Design review of the part built by this model. Coordinates are the model's own, in mm. A direction names the side the tool comes from. Give positions to 0.01 mm unless a question says otherwise; leave off trailing zeros. Order: outer loops, then holes, each group sorted by start corner. A loop starts at its lowest first (then second) coordinate and runs counter-clockwise, first axis right, second up. Notation, with made-up numbers: M 77,30.25 L 95,30.25 A11 cw 95,50.25 Z; hole C 12.5,20.25 d11. An arc over 180 degrees is marked long. Answer as a JSON object with one key per item and string values.
from build123d import *
from build123d.topology import SkipClean

# Parameters (mm, degrees)
SKETCH2_R           = 3.556
BOSS_EXTRUDE1_DEPTH = 0.254
CUT_EXTRUDE1_DEPTH  = 15.202896108
CUT_EXTRUDE2_DEPTH  = 15.331771344
FILLET1_R           = 0.396875


with BuildPart() as part:
    # Sketch1 → Base-Revolve (revolve)
    with BuildSketch(Plane.XY, mode=Mode.PRIVATE) as base_revolve_sk:
        Polygon((7.112, 0), (7.112, 8.69315), (5.08, 8.69315), (5.08, 8.1153), (3.556, 8.1153), (0, 8.1153), (0, 0), align=None)
    revolve(base_revolve_sk.sketch.rotate(Axis((0, 0, 0), (1, 0, 0)), 90), axis=Axis((0, 0, 0), (1, 0, 0)))

    # Sketch2 → Boss-Extrude1 (add)
    with BuildSketch(Plane(origin=(7.112, 0, 0), x_dir=(0, 0, -1), z_dir=(1, 0, 0))):
        with Locations(Location((0, 0, 0), (0, 0, 180))):
            Circle(SKETCH2_R)
    extrude(amount=BOSS_EXTRUDE1_DEPTH)

    # Sketch3 → Cut-Extrude1 (cut, through all)
    with SkipClean():  # the faces are left unmerged after this step: merging them gives an invalid solid
        with BuildSketch(Plane(origin=(7.112, 0, 0), x_dir=(0, 0, -1), z_dir=(1, 0, 0))):
            with BuildLine():
                ThreePointArc((2.61585906, -5.29454546), (5.9055, 0), (2.61585906, 5.29454546))
                ThreePointArc((2.61585906, 5.29454546), (1.042283968, 4.761688488), (1.57514094, 3.188113395))
                ThreePointArc((1.57514094, 3.188113395), (3.556, 0), (1.57514094, -3.188113395))
                ThreePointArc((1.57514094, -3.188113395), (1.042283968, -4.761688488), (2.61585906, -5.29454546))
            make_face()
            with BuildLine():
                ThreePointArc((-2.61585906, -5.29454546), (-1.042283968, -4.761688488), (-1.57514094, -3.188113395))
                ThreePointArc((-1.57514094, -3.188113395), (-3.556, 0), (-1.57514094, 3.188113395))
                ThreePointArc((-1.57514094, 3.188113395), (-1.042283968, 4.761688488), (-2.61585906, 5.29454546))
                ThreePointArc((-2.61585906, 5.29454546), (-5.9055, 0), (-2.61585906, -5.29454546))
            make_face()
        extrude(amount=-CUT_EXTRUDE1_DEPTH, mode=Mode.SUBTRACT)

    # Sketch4 → Cut-Extrude2 (cut, through all)
    with SkipClean():  # the faces are left unmerged after this step: merging them gives an invalid solid
        with BuildSketch(Plane(origin=(7.366, 0, 0), x_dir=(0, 0, -1), z_dir=(1, 0, 0))):
            with BuildLine():
                Line((3.434727855, 0.92075), (0.92075, 0.92075))
                Line((0.92075, 0.92075), (0.92075, 2.202919244))
                ThreePointArc((0.92075, 2.202919244), (0, 2.3876), (-0.92075, 2.202919244))
                Line((-0.92075, 2.202919244), (-0.92075, 0.92075))
                Line((-0.92075, 0.92075), (-3.434727855, 0.92075))
                ThreePointArc((-3.434727855, 0.92075), (-3.556, 0), (-3.434727855, -0.92075))
                Line((-3.434727855, -0.92075), (-0.92075, -0.92075))
                Line((-0.92075, -0.92075), (-0.92075, -2.202919244))
                ThreePointArc((-0.92075, -2.202919244), (0, -2.3876), (0.92075, -2.202919244))
                Line((0.92075, -2.202919244), (0.92075, -0.92075))
                Line((0.92075, -0.92075), (3.434727855, -0.92075))
                ThreePointArc((3.434727855, -0.92075), (3.556, 0), (3.434727855, 0.92075))
            make_face()
        extrude(amount=-CUT_EXTRUDE2_DEPTH, mode=Mode.SUBTRACT)

    # Fillet1
    fillet1_edges = [part.edges().sort_by_distance(p)[0] for p in [
        (3.683, -0.92075, -0.92075),
        (3.683, -0.92075, 0.92075),
        (3.683, 0.92075, 0.92075),
        (3.683, 0.92075, -0.92075),
    ]]
    fillet(fillet1_edges, radius=FILLET1_R)

    # Boss-Mirror1: part across face


with BuildPart() as part_1:
    with SkipClean():  # the faces are left unmerged after this step: merging them gives an invalid solid
        add(part.part)
        add(part.part.mirror(Plane.ZY))


solid = part_1.part
(1) We need section C-C (x = -2). Write out the cut boundary in (y, z), plus the area to 3 significant figures.
Checked values:
{"outline": "C 0,0 d16.23; hole M -5.29,-2.62 A5.91 ccw 5.29,-2.62 A1.17 ccw 3.19,-1.58 A3.56 cw 0.92,-3.43 L 0.92,-1.32 A0.4 cw 1.32,-0.92 L 2.2,-0.92 A2.39 ccw 2.2,0.92 L 1.32,0.92 A0.4 cw 0.92,1.32 L 0.92,3.43 A3.56 cw 3.19,1.58 A1.17 ccw 5.29,2.62 A5.91 ccw -5.29,2.62 A1.17 ccw -3.19,1.58 A3.56 cw -0.92,3.43 L -0.92,1.32 A0.4 cw -1.32,0.92 L -2.2,0.92 A2.39 ccw -2.2,-0.92 L -1.32,-0.92 A0.4 cw -0.92,-1.32 L -0.92,-3.43 A3.56 cw -3.19,-1.58 A1.17 ccw Z", "area": "131 mm^2"}
(2) Tool access review of faces 5 (the flat face through (0, 0.921, -2)), 6 (the flat face through (-5.08, 6, 6)), 7 (the flat face through (7.366, 3, 0)): name each direction out of +Z, -Z, +X, -X, +Y, -Y from which nothing blocks a thin tool from reaching the whole face with its end or side.
Checked values:
{"face 5": "+X, -X", "face 6": "none", "face 7": "+Z, -Z, +X, +Y, -Y"}
(3) Insertion check: pin 1 (4 mm diameter, centred on x = 0.5, y = -1.5, fed in from -Z); pin 2 (1.7 mm diameter, centred on x = -3, z = 2.5, fed in from -Y); pin 3 (4 mm diameter, centred on y = 5.5, z = -3.5, fed in from -X). Each pin has a flat end and moves straight along its axis. Give the tip position at first contact, or say it passes through.
Checked values:
{"pin 1": "stops at z = -8.12", "pin 2": "stops at y = -7.95", "pin 3": "stops at x = -7.11"}
(4) Draft analysis for pull direction X (two halves, no side actions). For faces 1 (the flat face through (7.112, 4, 0)), 2 (the flat face through (-7.112, 4, 0)), 3 (the cylindrical face through (0.07, 4.94, -6.44)), 4 (the flat face through (5.08, 6, 6)), state which applies: +X half, -X half, draft (parallel to the pull), parting line (faces both ways), or undercut.
Checked values:
{"face 1": "+X half", "face 2": "-X half", "face 3": "undercut", "face 4": "undercut"}
(5) To check wall thickness, follow L1, parallel to Y at x = -6, z = 2.25; L2, parallel to Z at x = -6.5, y = -4; L3, parallel to Z at x = -1.25, y = 3. State the ranges of each line that lie inside material, in increasing order. Write a range as from..to.
Checked values:
{"L1": "y = -8.4..-5.41, -2.75..-0.92, 0.92..2.75, 5.41..8.4", "L2": "z = -7.72..-4.34, -0.95..0.95, 4.34..7.72", "L3": "z = -7.54..-5.09, -1.91..1.91, 5.09..7.54"}
(6) We need section B-B (y = 0). Write out the cut boundary in (x, z).
Checked values:
{"outline": "M -7.11,-8.69 L -5.08,-8.69 L -5.08,-8.12 L 5.08,-8.12 L 5.08,-8.69 L 7.11,-8.69 L 7.11,-5.91 L -7.11,-5.91 Z; M -7.11,5.91 L 7.11,5.91 L 7.11,8.69 L 5.08,8.69 L 5.08,8.12 L -5.08,8.12 L -5.08,8.69 L -7.11,8.69 Z"}
(7) We need section A-A (z = 0). Write out the cut boundary in (x, y), plus the area to 3 significant figures.
Checked values:
{"outline": "M -7.37,-3.56 L -7.11,-3.56 L -7.11,-8.69 L -5.08,-8.69 L -5.08,-8.12 L 5.08,-8.12 L 5.08,-8.69 L 7.11,-8.69 L 7.11,-3.56 L 7.37,-3.56 L 7.37,-2.39 L -7.37,-2.39 Z; M -7.37,2.39 L 7.37,2.39 L 7.37,3.56 L 7.11,3.56 L 7.11,8.69 L 5.08,8.69 L 5.08,8.12 L -5.08,8.12 L -5.08,8.69 L -7.11,8.69 L -7.11,3.56 L -7.37,3.56 Z", "area": "169 mm^2"}
(8) We need section D-D (z = -2). Write out the cut boundary in (x, y) (3 decimals).
Checked values:
{"outline": "M -7.366,-2.94 L 7.366,-2.94 L 7.366,-0.921 L -7.366,-0.921 Z; M -7.366,0.921 L 7.366,0.921 L 7.366,2.94 L -7.366,2.94 Z; M -7.112,-8.46 L -5.08,-8.46 L -5.08,-7.865 L 5.08,-7.865 L 5.08,-8.46 L 7.112,-8.46 L 7.112,-5.412 L -7.112,-5.412 Z; M -7.112,5.412 L 7.112,5.412 L 7.112,8.46 L 5.08,8.46 L 5.08,7.865 L -5.08,7.865 L -5.08,8.46 L -7.112,8.46 Z"}
